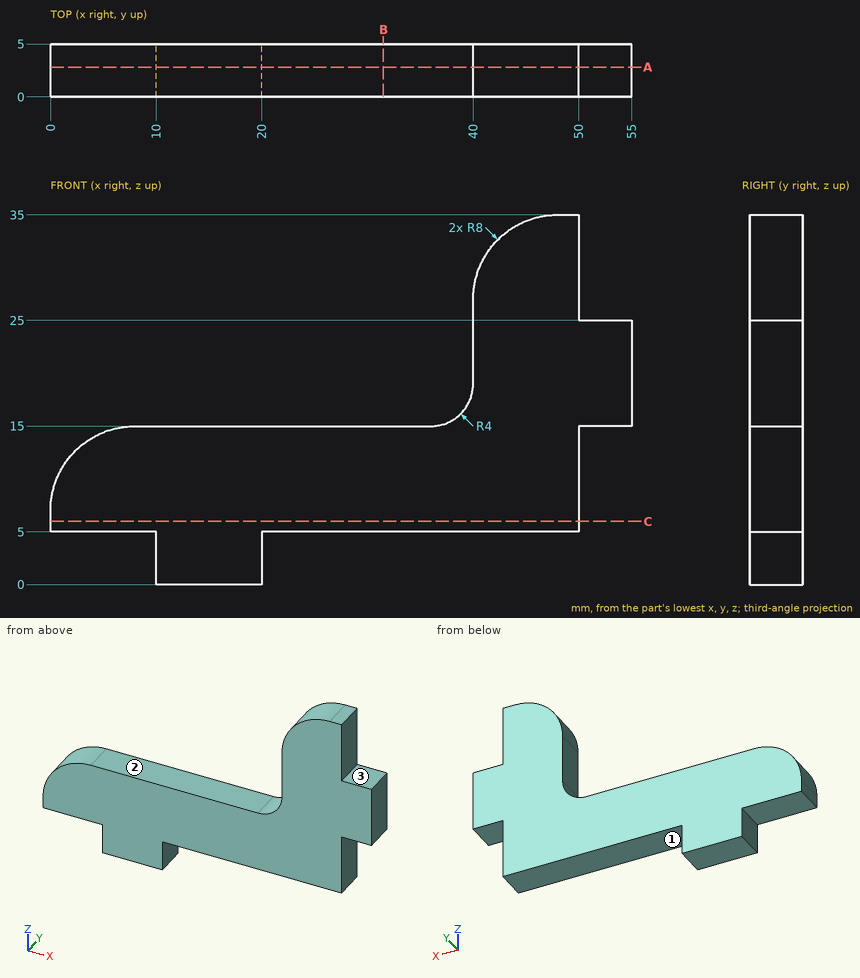
Design review of the part shown in the three views and the two pictorial views. Dimensions are in mm from the part's minimum x, y and z. A direction names the side the tool comes from. Round coordinates to 2 decimals unless told otherwise and drop trailing zeros. Loops run counter-clockwise (first coordinate to the right, second up) from the corner with the lowest first, then second, coordinate; pieces in that order, holes last. Notation, with made-up numbers: (-10, 62.5) - (41, 62.5) arc R21 cw to (41, 70.5) - close; hole circle Ø11 at (33.25, -37). An arc over 180 degrees is marked (long way). Write each question's results on one line, items separated by ' | '. Start each with the question number.
Q1. Take a section at C-C on z = 6. Give the boundary of the cut face in (x, y), plus the area to 3 significant figures.
Q2. Tool access review of the marked faces 1, 2 and 3: name each direction out of +Z, -Z, +X, -X, +Y, -Y from which nothing blocks a thin tool from reaching the whole face with its end or side.
Q3. Wall thickness on line 1 along X through (y, z) = (2.1, 3); line 2 along Z through (x, y) = (13, 0.35); line 3 along X through (y, z) = (4.7, 21): over which ranges is each line inside the solid? List them lowest first. Write a range as [from, to].
Q4. Take a section at A-A on y = 2.8. Give the boundary of the cut face in (x, z), plus the area to 3 significant figures.
Q5. Insertion check: P1, Ø2.5, axis at y = 2, z = 2.5, coming from the -X side; P2, Ø1.5, axis at x = 51.5, y = 2, coming from the +Z side; P3, Ø1.5, axis at y = 3, z = 8, coming from the +X side. Each pin has a flat end and moves straight along its axis. Give the tip position at first contact, or say it passes through.
Q6. Take a section at B-B on x = 31.5. Give the boundary of the cut face in (y, z), plus the area to 3 significant figures.
Data:
1) outline: (0, 0) - (50, 0) - (50, 5) - (0, 5) - close | area: 250 mm²
2) face 1: -Z, +X, +Y, -Y | face 2: +Z, -X, +Y, -Y | face 3: +Z, +X, +Y, -Y
3) line 1: x = [10, 20] | line 2: z = [0, 15] | line 3: x = [40, 55]
4) outline: (0, 5) - (10, 5) - (10, 0) - (20, 0) - (20, 5) - (50, 5) - (50, 15) - (55, 15) - (55, 25) - (50, 25) - (50, 35) - (48, 35) arc R8 ccw to (40, 27) - (40, 19) arc R4 cw to (36, 15) - (8, 15) arc R8 ccw to (0, 7) - close | area: 776 mm²
5) P1: stops at x = 10 | P2: stops at z = 25 | P3: stops at x = 50
6) outline: (0, 5) - (5, 5) - (5, 15) - (0, 15) - close | area: 50.0 mm²
